The listing builds one solid part. Answer for the finished solid, in the listing's coordinates (mm). A direction names the side the tool comes from. Coordinates: 2 decimals unless noted, no trailing zeros. Order: outer loops, then holes, each group sorted by start corner. A loop starts at its lowest first (then second) coordinate and runs counter-clockwise, first axis right, second up.
```python
from build123d import *

# Parameters (mm, degrees)
SKETCH1_W           = 23
SKETCH1_H           = 12
BOSS_EXTRUDE1_DEPTH = 20
BOSS_EXTRUDE2_DEPTH = 2
SKETCH3_W           = 23
SKETCH3_H           = 12
BOSS_EXTRUDE3_DEPTH = 2
BOSS_EXTRUDE4_DEPTH = 4.5
SKETCH5_R           = 2.75
BOSS_EXTRUDE5_DEPTH = 5
FILLET1_R           = 1


with BuildPart() as part:
    # Sketch1 → Boss-Extrude1 (new body)
    with BuildSketch(Plane(origin=(0, 0, 0), x_dir=(1, 0, 0), z_dir=(0, 1, 0))):
        Rectangle(SKETCH1_W, SKETCH1_H)
    extrude(amount=BOSS_EXTRUDE1_DEPTH)

    # Sketch2 → Boss-Extrude2 (add)
    with BuildSketch(Plane(origin=(0, 20, 0), x_dir=(1, 0, 0), z_dir=(0, 1, 0))):
        with BuildLine():
            Line((-16, 6), (16, 6))
            Line((16, 6), (16, 1.414213562))
            ThreePointArc((16, 1.414213562), (12.585786438, 0), (16, -1.414213562))
            Line((16, -1.414213562), (16, -6))
            Line((16, -6), (-16, -6))
            Line((-16, -6), (-16, -1.414213562))
            ThreePointArc((-16, -1.414213562), (-12.585786438, 0), (-16, 1.414213562))
            Line((-16, 1.414213562), (-16, 6))
        make_face()
    extrude(amount=BOSS_EXTRUDE2_DEPTH)

    # Sketch3 → Boss-Extrude3 (add)
    with BuildSketch(Plane(origin=(0, 22, 0), x_dir=(1, 0, 0), z_dir=(0, 1, 0))):
        Rectangle(SKETCH3_W, SKETCH3_H)
    extrude(amount=BOSS_EXTRUDE3_DEPTH)

    # Sketch4 → Boss-Extrude4 (add)
    with BuildSketch(Plane(origin=(0, 24, 0), x_dir=(1, 0, 0), z_dir=(0, 1, 0))):
        with BuildLine():
            ThreePointArc((-0.25, 2.90473751), (-11.5, 0), (-0.25, -2.90473751))
            ThreePointArc((-0.25, -2.90473751), (3.5, 0), (-0.25, 2.90473751))
        make_face()
    extrude(amount=BOSS_EXTRUDE4_DEPTH)

    # Sketch5 → Boss-Extrude5 (add)
    with BuildSketch(Plane(origin=(0, 28.5, 0), x_dir=(1, 0, 0), z_dir=(0, 1, 0))):
        with Locations(Location((-5.5, 0, 0), (0, 0, 270))):
            Circle(SKETCH5_R)
    extrude(amount=BOSS_EXTRUDE5_DEPTH)

    # Fillet1
    fillet1_edges = [part.edges().sort_by_distance(p)[0] for p in [
        (16, 21, 6),
        (16, 21, -6),
        (-16, 21, -6),
        (-16, 21, 6),
        (11.5, 23, 6),
        (11.5, 23, -6),
        (-11.5, 23, -6),
        (-11.5, 23, 6),
        (0, 0, 6),
        (-11.5, 0, 0),
        (0, 0, -6),
        (11.5, 0, 0),
        (11.5, 10, 6),
        (-11.5, 10, 6),
        (-11.5, 10, -6),
        (11.5, 10, -6),
    ]]
    fillet(fillet1_edges, radius=FILLET1_R)


solid = part.part
```
(1) Find section A-A (y = 14). Write down the section's boundary in (x, z).
(2) Each of these flat-tipped pins is pushed along its axis until it touches: pin 1 Ø1 at (y, z) = (23, 2) entering from -X; pin 2 Ø1 at (y, z) = (23, 0) entering from +X; pin 3 Ø3 at (x, z) = (14.5, 2) entering from +Y. Where does it stop, or does it pass through?
(3) Consider line 1 (Y direction, x = 3.5, z = -1); line 2 (Y direction, x = 1.5, z = -2.75); line 3 (X direction, y = 9, z = 1). Determine where each line is inside the solid, lowest interval first.
(4) Find section B-B (x = 0.5). Write down the section's boundary in (y, z).
(5) The mould has two halves that part along Z. Classify faces 1 (the face through (11.199, 10.633, -5.715)), 2 (the face through (-12.587, 20.986, 0.066)), 3 (the face through (-11.5, 23, 0)): released by +Z, released by -Z, zero draft, split by the parting line, or undercut.
(6) For faces 4 (the face through (-10, 24, -5)), 5 (the face through (-11.5, 10, 0)), 6 (the face through (-10, 24, 5)), 7 (the face through (3.5, 26.2, 0.1)), determine the directions among +Z, -Z, +X, -X, +Y, -Y from which every point of the face is accessible in a straight line to the end or side of a thin tool.
(7) Find section C-C (z = 3.5). Write down the section's boundary in (x, y).
(8) Find section D-D (y = 21). Write down the section's boundary in (x, z).
Findings below:
1. outline: (-11.5, -5) arc R1 ccw to (-10.5, -6) - (10.5, -6) arc R1 ccw to (11.5, -5) - (11.5, 5) arc R1 ccw to (10.5, 6) - (-10.5, 6) arc R1 ccw to (-11.5, 5) - close
2. pin 1: stops at x = -11.5
2. pin 2: stops at x = 11.5
2. pin 3: stops at y = 22
3. line 1: y = 0 to 24
3. line 2: y = 0 to 28.5
3. line 3: x = -11.5 to 11.5
4. outline: (0, -5) arc R1 ccw to (1, -6) - (24, -6) - (24, -3) - (28.5, -3) - (28.5, 3) - (24, 3) - (24, 6) - (1, 6) arc R1 ccw to (0, 5) - close
5. face 1: released by -Z
5. face 2: undercut
5. face 3: zero draft
6. face 4: -Z, -X, +Y
6. face 5: +Z, -Z, -X, -Y
6. face 6: +Z, -X, +Y
6. face 7: +Y
7. outline: (-16, 20) - (-11.5, 20) - (-11.5, 1) arc R1 ccw to (-10.5, 0) - (10.5, 0) arc R1 ccw to (11.5, 1) - (11.5, 20) - (16, 20) - (16, 22) - (11.5, 22) - (11.5, 24) - (-0.63, 24) - (-0.63, 28.5) - (-10.37, 28.5) - (-10.37, 24) - (-11.5, 24) - (-11.5, 22) - (-16, 22) - close
8. outline: (-16, -5) arc R1 ccw to (-15, -6) - (15, -6) arc R1 ccw to (16, -5) - (16, -1.41) arc R2 cw (long way) to (16, 1.41) - (16, 5) arc R1 ccw to (15, 6) - (-15, 6) arc R1 ccw to (-16, 5) - (-16, 1.41) arc R2 cw (long way) to (-16, -1.41) - close
